from build123d import *

# Parameters (mm, degrees)
SKETCH1_R           = 3
BOSS_EXTRUDE1_DEPTH = 27.5
SKETCH3_R           = 18
CUT_EXTRUDE1_DEPTH  = 1
SKETCH7_R           = 3
CUT_EXTRUDE2_DEPTH  = 20
SKETCH8_R           = 3
CUT_EXTRUDE3_DEPTH  = 16


with BuildPart() as part:
    # Sketch1 → Boss-Extrude1 (new body)
    with BuildSketch(Plane.XY):
        with BuildLine():
            Line((0, 40), (0, 5))
            ThreePointArc((0, 5), (-1.464466094, 1.464466094), (-5, 0))
            Line((-5, 0), (-40, 0))
            ThreePointArc((-40, 0), (-43.535533906, 1.464466094), (-45, 5))
            Line((-45, 5), (-45, 40))
            ThreePointArc((-45, 40), (-43.535533906, 43.535533906), (-40, 45))
            Line((-40, 45), (-5, 45))
            ThreePointArc((-5, 45), (-1.464466094, 43.535533906), (0, 40))
        make_face()
        with Locations((-6, 39)):
            Circle(SKETCH1_R, mode=Mode.SUBTRACT)
        with Locations((-6, 6)):
            Circle(SKETCH1_R, mode=Mode.SUBTRACT)
        with Locations((-39, 6)):
            Circle(SKETCH1_R, mode=Mode.SUBTRACT)
        with Locations((-39, 39)):
            Circle(SKETCH1_R, mode=Mode.SUBTRACT)
    extrude(amount=BOSS_EXTRUDE1_DEPTH)

    # Sketch3 → Cut-Extrude1 (cut)
    with BuildSketch(Plane.XY.offset(27.5)):
        with Locations((-22.5, 22.5)):
            Circle(SKETCH3_R)
    extrude(amount=-CUT_EXTRUDE1_DEPTH, mode=Mode.SUBTRACT)

    # Sketch7 → Cut-Extrude2 (cut)
    with BuildSketch(Plane(origin=(0, 45, 0), x_dir=(1, 0, 0), z_dir=(0, 1, 0))):
        with Locations((-22.5, -14)):
            Circle(SKETCH7_R)
    extrude(amount=-CUT_EXTRUDE2_DEPTH, mode=Mode.SUBTRACT)

    # Sketch8 → Cut-Extrude3 (cut)
    with BuildSketch(Plane.XY.offset(26.5)):
        with Locations((-22.5, 22.5)):
            Circle(SKETCH8_R)
    extrude(amount=-CUT_EXTRUDE3_DEPTH, mode=Mode.SUBTRACT)


solid = part.part
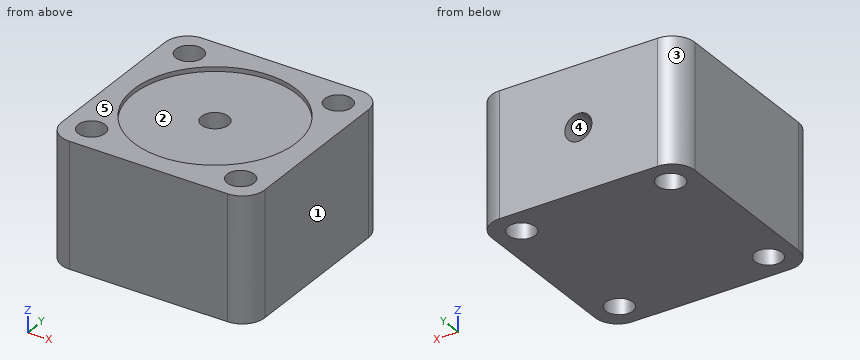
Verification items for the finished model (mm, model axes). Face numbers are marked on the shaded views. A direction names the side the tool comes from. Coordinates: 2 decimals unless noted, no trailing zeros. Order: outer loops, then holes, each group sorted by start corner. A loop starts at its lowest first (then second) coordinate and runs counter-clockwise, first axis right, second up. Notation, with made-up numbers: M 7,-30.75 L 43,-30.75 A30 ccw 43,7.25 Z; hole C 82,4 d3. An arc over 180 degrees is marked long. One line per item, written item: value. Start each with the question number.
Item 1: Sectioned sample at C-C on y = 6. Record the cut outline in (x, z).
Item 2: Mould release check, pull along X, two halves, no side actions. Record for the marked faces 3, 4 and 5: pulls with the +X half, pulls with the -X half, needs draft (parallel to the pull), parting line crosses it, or undercut.
Item 3: Sectioned sample at A-A on z = 8. Record the cut outline in (x, y).
Item 4: Sectioned sample at B-B on x = -39. Record the cut outline in (y, z).
Item 5: Thickness scan on probe 1 along Y at (x, z) = (-6, 11.25); probe 2 along Y at (x, z) = (-22.5, 23.75); probe 3 along Y at (x, z) = (-8.5, 22). Record the ranges inside material, lowest first.
Item 6: Depth check by flat-ended pin: P1, Ø21.5, axis at x = -22.5, y = 22.5, coming from the +Z side; P2, Ø1.8, axis at x = -21.5, y = 23.5, coming from the +Z side. Enter the tip coordinate at first touch or a pass-through.
Item 7: Access from +Z, -Z, +X, -X, +Y, -Y to the whole of each face (thin tool, end or side, straight path). Record for the marked faces 1 and 2.
Item 8: Sectioned sample at D-D on y = 21.5. Record the cut outline in (x, z).
Calculated:
1. outline: M -45,0 L -42,0 L -42,27.5 L -45,27.5 Z; M -36,0 L -9,0 L -9,27.5 L -15.31,27.5 L -15.31,26.5 L -29.69,26.5 L -29.69,27.5 L -36,27.5 Z; M -3,0 L 0,0 L 0,27.5 L -3,27.5 Z
2. face 3: pulls with the -X half
2. face 4: undercut
2. face 5: needs draft
3. outline: M -45,5 A5 ccw -40,0 L -5,0 A5 ccw 0,5 L 0,40 A5 ccw -5,45 L -40,45 A5 ccw -45,40 Z; hole C -39,6 d6; hole C -39,39 d6; hole C -6,6 d6; hole C -6,39 d6
4. outline: M 0,0 L 3,0 L 3,27.5 L 0,27.5 Z; M 9,0 L 36,0 L 36,27.5 L 29.69,27.5 L 29.69,26.5 L 15.31,26.5 L 15.31,27.5 L 9,27.5 Z; M 42,0 L 45,0 L 45,27.5 L 42,27.5 Z
5. probe 1: 0 to 3, 9 to 36, 42 to 45
5. probe 2: 0 to 19.5, 25.5 to 45
5. probe 3: 0 to 4.34, 7.66 to 37.34, 40.66 to 45
6. P1: z = 26.5
6. P2: z = 10.5
7. face 1: +Z, -Z, +X, +Y, -Y
7. face 2: +Z
8. outline: M -45,0 L 0,0 L 0,27.5 L -4.53,27.5 L -4.53,26.5 L -19.67,26.5 L -19.67,10.5 L -25.33,10.5 L -25.33,26.5 L -40.47,26.5 L -40.47,27.5 L -45,27.5 Z
